Verification items for the finished model (mm, model axes). Face numbers are marked on the shaded views. Give positions to 0.01 mm unless a question says otherwise; leave off trailing zeros. Loops run counter-clockwise (first coordinate to the right, second up) from the corner with the lowest first, then second, coordinate; pieces in that order, holes last. Notation, with made-up numbers: M -33,-37 L -15,-37 A20 cw -15,-30 Z; hole C 31.25,3.5 d7. An arc over 180 degrees is marked long. Use a Markdown table: item, result.
Autodesk Inventor part; units mm, degrees
ref_plane "YZ Plane" through (0, 0, 0) normal (1, 0, 0) x (0, 1, 0)
ref_plane "XZ Plane" through (0, 0, 0) normal (0, 1, 0) x (-1, 0, 0)
ref_plane "XY Plane" through (0, 0, 0) normal (0, 0, 1) x (1, 0, 0)
sketch "Sketch1" plane through (0, 0, 0) normal (0, 0, 1) x (1, 0, 0)
  line L0 (-20, 35) -> (20, 35)
  line L1 (20, 35) -> (20, -35)
  line L2 (20, -35) -> (-20, -35)
  line L3 (-20, -35) -> (-20, 35)
  point P0 (0, 0)
  point P1 (0, 35)
  point P2 (20, 0)
  dimension "d0" = 40
  dimension "d1" = 70
extrude "Extrusion1" add sketch "Sketch1" along normal mid plane 4
sketch "Sketch2" plane through (0, 0, 2) normal (0, 0, 1) x (1, 0, 0)
  circle A0 centre (0, 13.5) radius 12.5
  circle A1 centre (-15.5, 29) radius 1.6
  circle A2 centre (15.5, 29) radius 1.6
  circle A3 centre (15.5, -2) radius 1.6
  circle A4 centre (-15.5, -2) radius 1.6
  line L0 (-15.5, 29) -> (15.5, 29) construction
  line L1 (20, 35) -> (-20, 35)
  line L2 (-15.5, -2) -> (-15.5, 29) construction
  point P0 (0, 0)
  point P1 (0, 29)
  point P2 (-15.5, 13.5)
  dimension "d4" = 3.2
  dimension "d5" = 31
  dimension "d6" = 31
  dimension "d7" = 21.5
  dimension "d8" = 25
extrude "Extrusion2" cut sketch "Sketch2" against normal up to next
sketch "Sketch3" plane through (0, 0, 2) normal (0, 0, 1) x (1, 0, 0)
  arc A0 (-7.9, -24.8) -> (-12.1, -24.8) centre (-10, -24.8) ccw
  arc A1 (12.1, -24.8) -> (7.9, -24.8) centre (10, -24.8) ccw
  line L0 (-10, -24.8) -> (10, -24.8) construction
  arc A2 (-12.1, -29) -> (-7.9, -29) centre (-10, -29) ccw
  arc A3 (7.9, -29) -> (12.1, -29) centre (10, -29) ccw
  line L1 (-12.1, -29) -> (-12.1, -24.8)
  line L2 (-7.9, -24.8) -> (-7.9, -29)
  line L3 (7.9, -24.8) -> (7.9, -29)
  line L4 (12.1, -29) -> (12.1, -24.8)
  line L5 (-20, -35) -> (20, -35)
  point P0 (0, 0)
  point P1 (0, -24.8)
  dimension "d11" = 4.2
  dimension "d12" = 4.2
  dimension "d13" = 20
  dimension "d14" = 6
extrude "Extrusion3" cut sketch "Sketch3" against normal up to next
fillet "Fillet1" radius 3 4 edges at (-20, -35, 0) (20, -35, 0) (20, 35, 0) (-20, 35, 0)
equation "\"d6\" = d5"
properties part number "nema17-mount-bottom-z-axis-v2"
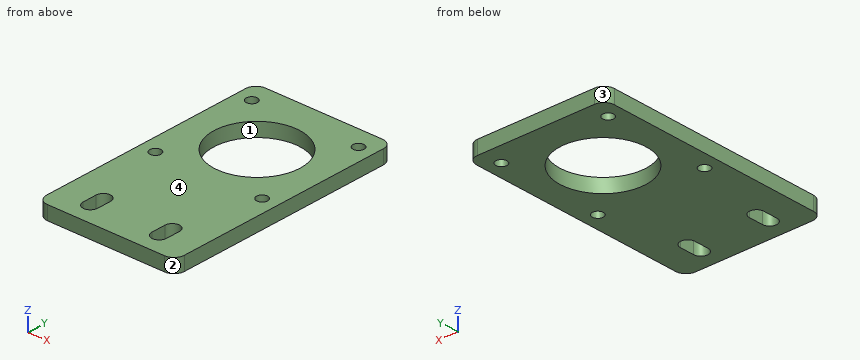
(1) Material ranges on line 1 (X direction, y = -25.5, z = -0.55); line 2 (Y direction, x = 9, z = 1.65); line 3 (Y direction, x = 9.5, z = 0.7), recorded low to high.
Results below:
| item | result |
|---|---|
| line 1 | -20 to -12.1, -7.9 to 7.9, 12.1 to 20 |
| line 2 | -35 to -30.85, -22.95 to 4.83, 22.17 to 35 |
| line 3 | -35 to -31.04, -22.76 to 5.38, 21.62 to 35 |
(2) Gauge pin test, flat end, axial feed: P1, Ø2.5, axis at x = -15.5, y = -2, coming from the +Z side. Record the tip position at first contact, or that the pin passes through.
Results below:
| item | result |
|---|---|
| P1 | through |
(3) Cross-section at B-B on x = 15.5. Record the cut outline in (y, z).
Results below:
| item | result |
|---|---|
| outline | M -35,-2 L -3.6,-2 L -3.6,2 L -35,2 Z; M -0.4,-2 L 27.4,-2 L 27.4,2 L -0.4,2 Z; M 30.6,-2 L 35,-2 L 35,2 L 30.6,2 Z |
(4) Draft check along Y on the marked faces 1, 2, 3 and 4. Enter one of: +Y half, -Y half, draft (parallel to the pull), parting line (faces both ways), or undercut.
Results below:
| item | result |
|---|---|
| face 1 | undercut |
| face 2 | -Y half |
| face 3 | +Y half |
| face 4 | draft |
(5) Cross-section at C-C on z = -0.2. Record the cut outline in (x, y).
Results below:
| item | result |
|---|---|
| outline | M -20,-32 A3 ccw -17,-35 L 17,-35 A3 ccw 20,-32 L 20,32 A3 ccw 17,35 L -17,35 A3 ccw -20,32 Z; hole C -15.5,-2 d3.2; hole C -15.5,29 d3.2; hole C 0,13.5 d25; hole M -12.1,-29 A2.1 ccw -7.9,-29 L -7.9,-24.8 A2.1 ccw -12.1,-24.8 Z; hole M 7.9,-29 A2.1 ccw 12.1,-29 L 12.1,-24.8 A2.1 ccw 7.9,-24.8 Z; hole C 15.5,-2 d3.2; hole C 15.5,29 d3.2 |
(6) Cross-section at D-D on x = 0. Record the cut outline in (y, z), then the cut area to 3 significant figures.
Results below:
| item | result |
|---|---|
| outline | M -35,-2 L 1,-2 L 1,2 L -35,2 Z; M 26,-2 L 35,-2 L 35,2 L 26,2 Z |
| area | 180 mm^2 |
(7) Cross-section at A-A on y = 13.5. Record the cut outline in (x, z).
Results below:
| item | result |
|---|---|
| outline | M -20,-2 L -12.5,-2 L -12.5,2 L -20,2 Z; M 12.5,-2 L 20,-2 L 20,2 L 12.5,2 Z |
